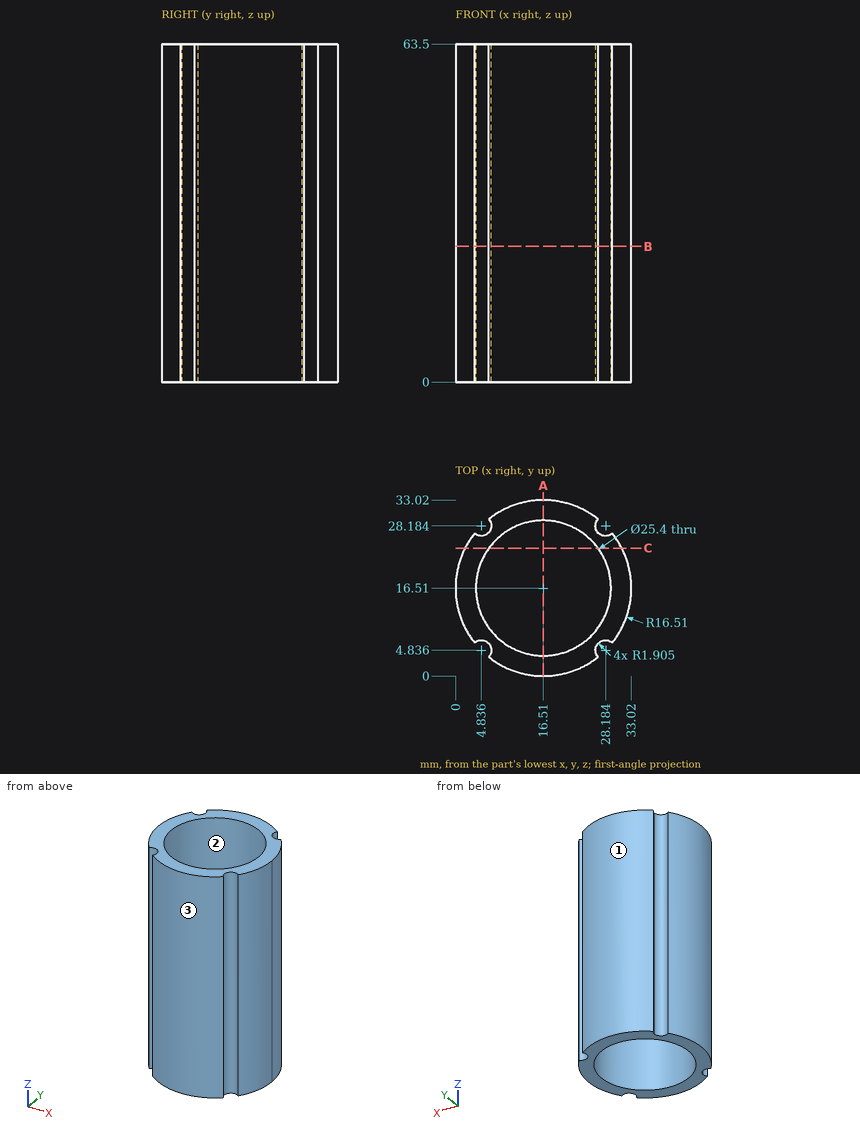
Could you check a few things on this drawing? It's one solid part, dimensions in mm from its lowest x, y, z. Give positions to 0.01 mm unless a question says otherwise; leave off trailing zeros. Order: outer loops, then holes, each group sorted by start corner. A loop starts at its lowest first (then second) coordinate and runs counter-clockwise, first axis right, second up. Notation, with made-up numbers: (1, 28) - (10, 28) arc R18 ccw to (10, 51) - close; hole circle Ø7 at (-8, 43). An arc over 180 degrees is marked (long way). One line per item, written item: value. Start each with the question number.
1. Imagine slicing it at A-A on x = 16.5. List the corners of the cut face in (y, z) for me, plus the area to 3 significant figures.
2. Thinking about a two-plate mould opening in Y: for the marked faces 1, 2 and 3, which applies, +Y half, -Y half, draft (parallel to the pull), parting line (faces both ways), or undercut?
3. Imagine slicing it at B-B on z = 25.5. List the corners of the cut face in (x, y) for me (1 decimal).
4. Imagine slicing it at C-C on y = 24. List the corners of the cut face in (x, z) for me, plus the area to 3 significant figures.
5. For P1, Ø5, axis at x = 8, z = 31, coming from the -Y side; P2, Ø12, axis at y = 10, z = 25.5, coming from the -X side; P3, Ø8, axis at x = 21, z = 20, coming from the +Y side; P4, Ø8, axis at x = 12, y = 28, coming from the -Z side, each with a flat end and sliding along its axis, tell me the tip position at first contact or that it passes through.
6. If I drill on probe 1 along Y at (x, z) = (16.51, 25); probe 2 along X at (y, z) = (16, 33); probe 3 along Y at (x, z) = (10.5, 38), over which ranges is the centre line in solid material (lowest first)?
Values:
1. outline: (0, 0) - (3.81, 0) - (3.81, 63.5) - (0, 63.5) - close; (29.21, 0) - (33.02, 0) - (33.02, 63.5) - (29.21, 63.5) - close
1. area: 484 mm²
2. face 1: +Y half
2. face 2: undercut
2. face 3: -Y half
3. outline: (3.6, 6.3) arc R1.9 cw to (6.7, 4.8) arc R1.9 cw to (6.3, 3.6) arc R16.5 ccw to (26.8, 3.6) arc R1.9 cw to (29.5, 6.3) arc R16.5 ccw to (33, 16.5) arc R16.5 ccw to (29.5, 26.8) arc R1.9 cw to (26.8, 29.5) arc R16.5 ccw to (6.3, 29.5) arc R1.9 cw to (6.7, 28.2) arc R1.9 cw to (3.6, 26.8) arc R16.5 ccw to start; hole circle Ø25.4 at (16.5, 16.5)
4. outline: (1.8, 0) - (6.25, 0) - (6.25, 63.5) - (1.8, 63.5) - close; (26.77, 0) - (31.22, 0) - (31.22, 63.5) - (26.77, 63.5) - close
4. area: 566 mm²
5. P1: y = 1.13
5. P2: x = 0.01
5. P3: y = 33.01
5. P4: z = 0
6. probe 1: 0 to 3.81, 29.21 to 33.02
6. probe 2: 0.01 to 3.82, 29.2 to 33.01
6. probe 3: 1.13 to 5.32, 27.7 to 31.89
